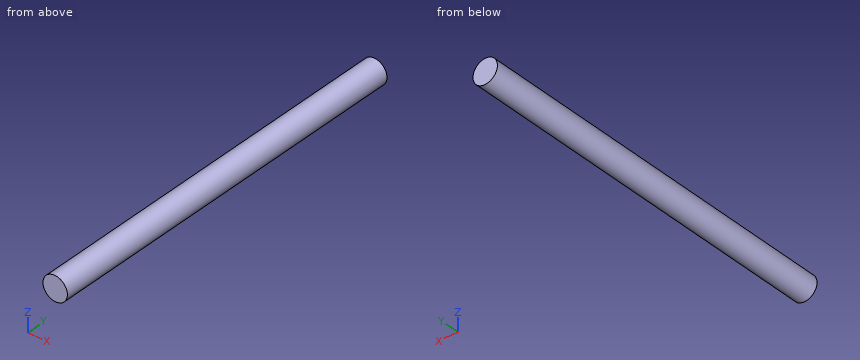
from build123d import *

# Parameters (mm, degrees)
F0_R     = 5.25
F1_DEPTH = 110
F2_DEPTH = 100
F3_DEPTH = 50


with BuildPart() as f1:
    # F0 (on Front) → F1 (new body)
    with BuildSketch(Plane.XZ):
        Circle(F0_R)
    extrude(amount=F1_DEPTH)

    # F2 (add): a face of the model
    f2_faces = [f1.faces().sort_by_distance(p)[0] for p in [
        (0, -110, 0),
    ]]
    extrude(f2_faces, amount=F2_DEPTH)

    # F3 (cut): a face of the model
    f3_faces = [f1.faces().sort_by_distance(p)[0] for p in [
        (0, -210, 0),
    ]]
    extrude(f3_faces, amount=-F3_DEPTH, mode=Mode.SUBTRACT)


solid = f1.part
For this review, take the finished solid that the model builds, in its own axes (mm). Round coordinates to 2 decimals unless told otherwise and drop trailing zeros. Order: outer loops, then holes, each group sorted by start corner. A loop starts at its lowest first (then second) coordinate and runs counter-clockwise, first axis right, second up. Notation, with made-up numbers: (32, 55) -> (91, 55) arc R27 cw to (91, 87) -> close; hole circle Ø3 at (-2, -22.5). An arc over 180 degrees is marked (long way). Put each result on its own line as item: value.
Q1. Add section A-A on y = -103. Write out the cut boundary in (x, z).
Check result:
outline: circle Ø10.5 at (0, 0)
Q2. Add section B-B on x = 3.25. Write out the cut boundary in (y, z).
Check result:
outline: (-160, -4.12) -> (0, -4.12) -> (0, 4.12) -> (-160, 4.12) -> close
Q3. Add section C-C on x = -2.75. Write out the cut boundary in (y, z), plus the area to 3 significant figures.
Check result:
outline: (-160, -4.47) -> (0, -4.47) -> (0, 4.47) -> (-160, 4.47) -> close
area: 1,430 mm2
Q4. Insertion check: pin 1 Ø1 at (y, z) = (-50, -2.5) entering from +X; pin 2 Ø1.5 at (x, z) = (3, 4) entering from +Y; pin 3 Ø6 at (y, z) = (-55.5, -4) entering from +X. Each pin has a flat end and moves straight along its axis. Give the tip position at first contact, or say it passes through.
Check result:
pin 1: x = 4.85
pin 2: y = 0
pin 3: x = 5.15
Q5. For probe 1 along Z at (x, y) = (-0.25, -127.5); probe 2 along X at (y, z) = (-59, 1.5); probe 3 along Z at (x, y) = (-2, -150), list the stretches that pass through material, from the lowest coordinate up. Write a range as [from, to].
Check result:
probe 1: [-5.24, 5.24]
probe 2: [-5.03, 5.03]
probe 3: [-4.85, 4.85]
